Source: CAD feature listing. Evaluate the final solid. Frame: model axes, mm. A direction names the side the tool comes from. Give positions to 0.01 mm unless a question says otherwise; leave off trailing zeros. Write each loop counter-clockwise with the first axis right and the second up, starting at its lowest first coordinate (ties: lowest second). Pieces come first, ordered by that corner, then holes. Notation, with made-up numbers: M 21,9.5 L 73,9.5 A10 ccw 73,28.5 Z; hole C 20.25,-13 d6. An arc over 180 degrees is marked long. Return JSON: item names as keys, results as strings.
```python
from build123d import *

# Parameters (mm, degrees)
SKETCH2_W           = 40
SKETCH2_H           = 20
BOSS_EXTRUDE1_DEPTH = 37
SKETCH3_W           = 20
SKETCH3_H           = 2.5
BOSS_EXTRUDE2_DEPTH = 7
SKETCH4_R           = 2.5
CUT_EXTRUDE5_DEPTH  = 7.25
SKETCH5_R           = 2.75
BOSS_EXTRUDE4_DEPTH = 7.1
FILLET1_R           = 2
FILLET2_R           = 1


with BuildPart() as part:
    # Sketch2 → Boss-Extrude1 (new body)
    with BuildSketch(Plane(origin=(0, 0, 0), x_dir=(1, 0, 0), z_dir=(0, 1, 0))):
        with Locations((20, 10)):
            Rectangle(SKETCH2_W, SKETCH2_H)
    extrude(amount=BOSS_EXTRUDE1_DEPTH)

    # Sketch3 → Boss-Extrude2 (add)
    with BuildSketch(Plane.ZY):
        with Locations((-10, 27.45)):
            Rectangle(SKETCH3_W, SKETCH3_H)
    boss_extrude2 = extrude(amount=BOSS_EXTRUDE2_DEPTH)

    # Mirror1: Boss-Extrude2 across plane
    add(boss_extrude2.mirror(Plane.ZY.offset(-20)))

    # Sketch4 → Cut-Extrude5 (cut)
    with BuildSketch(Plane(origin=(0, 28.7, 0), x_dir=(1, 0, 0), z_dir=(0, 1, 0))):
        with Locations((-4.75, 15)):
            Circle(SKETCH4_R)
        with Locations((-4.75, 5)):
            Circle(SKETCH4_R)
        with Locations((44.75, 5)):
            Circle(SKETCH4_R)
        with Locations((44.75, 15)):
            Circle(SKETCH4_R)
    extrude(amount=-CUT_EXTRUDE5_DEPTH, mode=Mode.SUBTRACT)

    # Sketch5 → Boss-Extrude4 (add)
    with BuildSketch(Plane(origin=(0, 37, 0), x_dir=(1, 0, 0), z_dir=(0, 1, 0))):
        with Locations(Location((29.9, 10, 0), (0, 0, 90))):
            Circle(SKETCH5_R)
    extrude(amount=BOSS_EXTRUDE4_DEPTH)

    # Fillet1
    fillet1_edges = [part.edges().sort_by_distance(p)[0] for p in [
        (20, 37, -20),
        (20, 0, -20),
        (20, 0, 0),
        (20, 37, 0),
    ]]
    fillet(fillet1_edges, radius=FILLET1_R)

    # Fillet2
    fillet2_edges = [part.edges().sort_by_distance(p)[0] for p in [
        (0, 31.85, -20),
        (0, 36.414213562, -19.414213562),
        (0, 36.414213562, -0.585786438),
        (40, 0, -10),
        (40, 0.585786438, -19.414213562),
        (40, 0.585786438, -0.585786438),
        (0, 0, -10),
        (0, 0.585786438, -19.414213562),
        (0, 0.585786438, -0.585786438),
        (0, 14.1, 0),
        (0, 14.1, -20),
        (-7, 27.45, -20),
        (-7, 27.45, 0),
        (40, 14.1, -20),
        (40, 14.1, 0),
        (47, 27.45, -20),
        (47, 27.45, 0),
        (0, 37, -10),
        (40, 37, -10),
        (40, 31.85, 0),
        (40, 31.85, -20),
        (40, 36.414213562, -19.414213562),
        (40, 36.414213562, -0.585786438),
        (0, 31.85, 0),
    ]]
    fillet(fillet2_edges, radius=FILLET2_R)


solid = part.part
```
1) Cut plane C-C, the plane x = 14. Return the cut outline in (y, z).
Numbers:
{"outline": "M 0,-18 A2 ccw 2,-20 L 35,-20 A2 ccw 37,-18 L 37,-2 A2 ccw 35,0 L 2,0 A2 ccw 0,-2 Z"}
2) Contact query for flat-ended pins moving along their axis: pin 1 Ø9 at (y, z) = (20, -7) entering from +X; pin 2 Ø3 at (x, z) = (-1, -10) entering from +Y; pin 3 Ø4 at (x, z) = (9, -16.5) entering from +Y; pin 4 Ø2.5 at (x, z) = (-5, -14.5) entering from -Y. Output: stop coordinate, or through.
Numbers:
{"pin 1": "stops at x = 40", "pin 2": "stops at y = 36.87", "pin 3": "stops at y = 37", "pin 4": "passes through"}
3) Cut plane D-D, the plane z = -5. Return the cut outline in (x, y).
Numbers:
{"outline": "M -2.25,26.2 L 0,26.2 L 0,1 A1 ccw 1,0 L 39,0 A1 ccw 40,1 L 40,26.2 L 42.25,26.2 L 42.25,28.7 L 40,28.7 L 40,36 A1 ccw 39,37 L 1,37 A1 ccw 0,36 L 0,28.7 L -2.25,28.7 Z"}
4) Draft query along X for faces 6 (the face through (47, 27, -2)), 7 (the face through (43, 28.7, -10)), 8 (the face through (42.25, 27.47, -5.09)), 9 (the face through (42.25, 27.47, -15.09)). Return one class per face: released by +X, released by -X, zero draft, split by the parting line, or undercut.
Numbers:
{"face 6": "released by +X", "face 7": "zero draft", "face 8": "undercut", "face 9": "undercut"}
5) Set-up query: faces 1 (the face through (47, 27, -10)), 2 (the face through (20.27, 0.57, -0.6)), 3 (the face through (40, 13, -10)), 4 (the face through (0, 32, -10)), 5 (the face through (0, 13, -10)). Return all of +Z, -Z, +X, -X, +Y, -Y with unobstructed straight access to the full face (end or side cutting, diameter ignored); none if empty.
Numbers:
{"face 1": "+Z, -Z, +X, +Y, -Y", "face 2": "+Z, +X, -X, -Y", "face 3": "+Z, -Z, +X, -Y", "face 4": "+Z, -Z, -X, +Y", "face 5": "+Z, -Z, -X, -Y"}
6) Line query: line 1 (Z direction, x = -4.75, y = 27.8); line 2 (Z direction, x = 44, y = 27); line 3 (Y direction, x = -2, z = -7.5). Output: solid intervals per line, ascending. Write a range as [from, to].
Numbers:
{"line 1": "z = [-20, -17.5], [-12.5, -7.5], [-2.5, 0]", "line 2": "z = [-20, -17.38], [-12.62, -7.38], [-2.62, 0]", "line 3": "y = [26.2, 28.7]"}
7) Cut plane A-A, the plane x = -4.75. Return the cut outline in (y, z).
Numbers:
{"outline": "M 26.2,-20 L 28.7,-20 L 28.7,-17.5 L 26.2,-17.5 Z; M 26.2,-12.5 L 28.7,-12.5 L 28.7,-7.5 L 26.2,-7.5 Z; M 26.2,-2.5 L 28.7,-2.5 L 28.7,0 L 26.2,0 Z"}
8) Cut plane B-B, the plane y = 24.5. Return the cut outline in (x, z).
Numbers:
{"outline": "M 0,-19 A1 ccw 1,-20 L 39,-20 A1 ccw 40,-19 L 40,-1 A1 ccw 39,0 L 1,0 A1 ccw 0,-1 Z"}
